Read the model definition and answer for the solid it produces. Units are mm, in the model's axes. Face numbers are marked on the shaded views. A direction names the side the tool comes from. Coordinates: 2 decimals unless noted, no trailing zeros. Loops run counter-clockwise (first coordinate to the right, second up) from the corner with the lowest first, then second, coordinate; pieces in that order, holes last. Notation, with made-up numbers: M -24,-17.75 L 30,-17.75 A28 cw 30,11.25 Z; hole C 52,-19 d6. An arc over 180 degrees is marked long. Put each result on its own line as item: value.
from build123d import *

# Parameters (mm, degrees)
F0_R     = 60
F0_R_2   = 3
F0_R_3   = 15
F0_R_4   = 2
F1_DEPTH = 25


# Not quite as in the source:
# - a feature names something its author has since deleted; it is built from what else it names


with BuildPart() as f1:
    # F0 (on Front) → F1 (new body)
    with BuildSketch(Plane.XZ):
        Circle(F0_R)
        with Locations((-37.5115520048, -38.8443492183)):
            Circle(F0_R_2, mode=Mode.SUBTRACT)
        with BuildLine():
            ThreePointArc((-17.9991214641, -21.8181490168), (-12.909542723, -18.5322896083), (-6.8568272685, -18.7878662921))
            ThreePointArc((-6.8568272685, -18.7878662921), (0.003827401, -19.9999996338), (6.864017636, -18.7852405333))
            ThreePointArc((6.864017636, -18.7852405333), (12.9220689894, -18.5288245474), (18.0146364939, -21.8199476948))
            Line((18.0146364939, -21.8199476948), (27.2720618955, -33.0586128775))
            ThreePointArc((27.2720618955, -33.0586128775), (29.3324432338, -41.5072979988), (23.9974181864, -48.3748273422))
            ThreePointArc((23.9974181864, -48.3748273422), (0, -54), (-23.9974181864, -48.3748273422))
            ThreePointArc((-23.9974181864, -48.3748273422), (-29.3332198415, -41.5036623321), (-27.2673324169, -33.0528755612))
            Line((-27.2673324169, -33.0528755612), (-17.9991214641, -21.8181490168))
        make_face(mode=Mode.SUBTRACT)
        with BuildLine():
            ThreePointArc((-44.5250909536, -30.5534985815), (-45.2912230512, -29.4058687089), (-46.0277820813, -28.2390381684))
            ThreePointArc((-46.0277820813, -28.2390381684), (-46.5604522686, -23.0733436974), (-42.8629692739, -19.4268719232))
            Line((-42.8629692739, -19.4268719232), (-16.9967316552, -10.5409256254))
            ThreePointArc((-16.9967316552, -10.5409256254), (-15.120110809, -11.5154453431), (-15.5299138764, -13.5899226089))
            Line((-15.5299138764, -13.5899226089), (-16.9726013847, -14.8870728677))
            Line((-16.9726013847, -14.8870728677), (-17.1078816805, -15.0240893401))
            Line((-17.1078816805, -15.0240893401), (-35.5662381193, -31.6203804252))
            ThreePointArc((-35.5662381193, -31.6203804252), (-40.2873666152, -33.116567588), (-44.5250909536, -30.5534985815))
        make_face(mode=Mode.SUBTRACT)
        with Locations((-52.3959692189, -13.0637823624)):
            Circle(F0_R_2, mode=Mode.SUBTRACT)
        with Locations((37.5115520048, -38.8443492183)):
            Circle(F0_R_2, mode=Mode.SUBTRACT)
        with BuildLine():
            Line((21.3985322272, -7.6356383993), (45.0061435827, -15.3247300238))
            ThreePointArc((45.0061435827, -15.3247300238), (48.6715278542, -18.6865524369), (48.5414946952, -23.6584719025))
            ThreePointArc((48.5414946952, -23.6584719025), (46.8021183332, -26.9362528857), (44.8417435514, -30.0868415635))
            ThreePointArc((44.8417435514, -30.0868415635), (40.6476491874, -32.6918461445), (35.9197630861, -31.2693239428))
            Line((35.9197630861, -31.2693239428), (17.1994124126, -14.9726488191))
            ThreePointArc((17.1994124126, -14.9726488191), (16.1962922773, -13.1122239789), (16.6688649306, -11.0521012448))
            ThreePointArc((16.6688649306, -11.0521012448), (17.2612476069, -10.1019468943), (17.7995287636, -9.1201302509))
            ThreePointArc((17.7995287636, -9.1201302509), (19.3255292381, -7.7148076154), (21.3985322272, -7.6356383993))
        make_face(mode=Mode.SUBTRACT)
        with Locations((52.3959692189, -13.0637823624)):
            Circle(F0_R_2, mode=Mode.SUBTRACT)
        with BuildLine():
            Line((-14.9909636957, 40.1406403471), (-9.8955105801, 26.4967709421))
            ThreePointArc((-9.8955105801, 26.4967709421), (-9.5946622296, 20.4461367535), (-12.8423558576, 15.3321197499))
            ThreePointArc((-12.8423558576, 15.3321197499), (-18.0436420311, 8.6271074095), (-19.9965959104, 0.3689877998))
            ThreePointArc((-19.9965959104, 0.3689877998), (-22.4237136521, -5.9792994979), (-28.3480846215, -9.3099872294))
            Line((-28.3480846215, -9.3099872294), (-42.3172195747, -11.6422803342))
            ThreePointArc((-42.3172195747, -11.6422803342), (-50.2710809676, -9.5390364788), (-53.9558535504, -2.1830867246))
            ThreePointArc((-53.9558535504, -2.1830867246), (-48.0998424018, 24.5439434672), (-29.8951202889, 44.9697874457))
            ThreePointArc((-29.8951202889, 44.9697874457), (-21.276616009, 46.1551447236), (-14.9909636957, 40.1406403471))
        make_face(mode=Mode.SUBTRACT)
        with BuildLine():
            Line((-4.4279652677, 22.3694685585), (-9.2474940163, 46.7170617057))
            ThreePointArc((-9.2474940163, 46.7170617057), (-8.1285920064, 51.5258593406), (-3.7819096653, 53.8674034949))
            ThreePointArc((-3.7819096653, 53.8674034949), (-0.1220878193, 53.9998619865), (3.5382955571, 53.8839536834))
            ThreePointArc((3.5382955571, 53.8839536834), (7.9230697986, 51.5261035304), (9.0182868498, 46.6695407434))
            Line((9.0182868498, 46.6695407434), (3.9392668723, 22.3644794699))
            ThreePointArc((3.9392668723, 22.3644794699), (2.8434498256, 20.6092434876), (0.8719123918, 19.9809851804))
            ThreePointArc((0.8719123918, 19.9809851804), (-0.2100325239, 19.9988971281), (-1.2913626084, 19.9582660222))
            ThreePointArc((-1.2913626084, 19.9582660222), (-3.31345185, 20.5735591973), (-4.4279652677, 22.3694685585))
        make_face(mode=Mode.SUBTRACT)
        with Locations((-14.8844172141, 51.9081315807)):
            Circle(F0_R_2, mode=Mode.SUBTRACT)
        Circle(F0_R_3, mode=Mode.SUBTRACT)
        with BuildLine():
            ThreePointArc((12.8423558576, 15.3321197499), (9.5946622296, 20.4461367535), (9.8955105801, 26.4967709421))
            Line((9.8955105801, 26.4967709421), (14.9909636957, 40.1406403471))
            ThreePointArc((14.9909636957, 40.1406403471), (21.276616009, 46.1551447236), (29.8951202889, 44.9697874457))
            ThreePointArc((29.8951202889, 44.9697874457), (46.7619600734, 27.0059084294), (53.8916763243, 3.4186580637))
            ThreePointArc((53.8916763243, 3.4186580637), (50.6128315094, -4.6370491105), (42.2649270201, -7.0778956919))
            Line((42.2649270201, -7.0778956919), (27.9019654451, -4.6798491157))
            ThreePointArc((27.9019654451, -4.6798491157), (22.506844055, -1.9164656047), (19.6991831261, 3.4557465422))
            ThreePointArc((19.6991831261, 3.4557465422), (17.3205080757, 10), (12.8423558576, 15.3321197499))
        make_face(mode=Mode.SUBTRACT)
        with Locations((14.8844172141, 51.9081315807)):
            Circle(F0_R_2, mode=Mode.SUBTRACT)
        Circle(F0_R_3)
        with Locations((-5.8778525229, -8.0901699437)):
            Circle(F0_R_4, mode=Mode.SUBTRACT)
        with BuildLine():
            ThreePointArc((-3.8729833462, 1), (-2.8284271247, 2.8284271247), (-1, 3.8729833462))
            Line((-1, 3.8729833462), (-1, 5))
            ThreePointArc((-1, 5), (0, 6), (1, 5))
            Line((1, 5), (1, 3.8729833462))
            ThreePointArc((1, 3.8729833462), (2.8284271247, 2.8284271247), (3.8729833462, 1))
            Line((3.8729833462, 1), (4.9514505081, 1))
            ThreePointArc((4.9514505081, 1), (5.9514505081, 0), (4.9514505081, -1))
            Line((4.9514505081, -1), (3.8729833462, -1))
            ThreePointArc((3.8729833462, -1), (2.8284271247, -2.8284271247), (1, -3.8729833462))
            Line((1, -3.8729833462), (1, -5.0126444548))
            ThreePointArc((1, -5.0126444548), (0, -6.0126444548), (-1, -5.0126444548))
            Line((-1, -5.0126444548), (-1, -3.8729833462))
            ThreePointArc((-1, -3.8729833462), (-2.8284271247, -2.8284271247), (-3.8729833462, -1))
            Line((-3.8729833462, -1), (-5.0453338772, -1))
            ThreePointArc((-5.0453338772, -1), (-6.0453338772, 0), (-5.0453338772, 1))
            Line((-5.0453338772, 1), (-3.8729833462, 1))
        make_face(mode=Mode.SUBTRACT)
        with Locations((5.8778525229, -8.0901699437)):
            Circle(F0_R_4, mode=Mode.SUBTRACT)
        with Locations((-9.510565163, 3.0901699437)):
            Circle(F0_R_4, mode=Mode.SUBTRACT)
        with Locations((9.510565163, 3.0901699437)):
            Circle(F0_R_4, mode=Mode.SUBTRACT)
        with Locations((0, 10)):
            Circle(F0_R_4, mode=Mode.SUBTRACT)
    extrude(amount=F1_DEPTH)


solid = f1.part
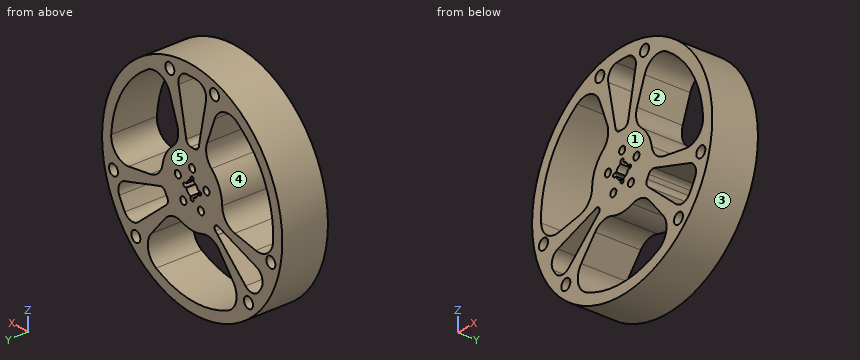
1) Which of the six approach directions +Z, -Z, +X, -X, +Y, -Y give full straight-line access (tool end or side, diameter ignored) to the marked faces 4 and 5?
Answer list:
face 4: +Y, -Y
face 5: +Z, -Z, +X, -X, +Y
2) Determine the mould class of the marked faces 1, 2 and 3 for opening direction X: released by +X, released by -X, zero draft, split by the parting line, or undercut.
Answer list:
face 1: zero draft
face 2: undercut
face 3: split by the parting line
3) Find section A-A, the plane z = 10. Write down the section's boundary in (x, y).
Answer list:
outline: M -59.16,-25 L -53.07,-25 L -53.07,0 L -59.16,0 Z; M -17.32,-25 L -2,-25 L -2,0 L -17.32,0 Z; M 2,-25 L 17.32,-25 L 17.32,0 L 2,0 Z; M 53.07,-25 L 59.16,-25 L 59.16,0 L 53.07,0 Z
4) Given pin 1 Ø1.3 at (y, z) = (-11, -4.5) entering from +X; pin 2 Ø3 at (x, y) = (-27, -21.5) entering from -Z; pin 3 Ø0.6 at (y, z) = (-15, -4.5) entering from -X; pin 4 Ø1 at (x, z) = (-12.5, 14.5) entering from +Y, each flat-ended and moving along its own axis, determine where each tip first touches the part or whether it passes through.
Answer list:
pin 1: stops at x = 59.88
pin 2: stops at z = -54.31
pin 3: stops at x = -59.85
pin 4: stops at y = 0
5) Straight lines are drawn through the part: line 1 (Z direction, x = -15.5, y = -5); line 2 (Z direction, x = 46.5, y = -17.75); line 3 (Z direction, x = 43.5, y = -18.25). For each, find the intervals that lie inside material, in ascending order. Write a range as [from, to].
Answer list:
line 1: z = [-57.96, -51.73], [-19.65, -13.56], [-11, 12.64], [41.28, 48.97], [54.84, 57.96]
line 2: z = [-37.92, -27.45], [-16.05, -6.87], [27.45, 37.92]
line 3: z = [-41.32, -31.51], [-14.83, -7.21], [32, 41.32]
6) Find section B-B, the plane y = -6.5. Count the separate pieces of the cut face and the enclosed holes in it, plus the area to 3 significant figures.
Answer list:
separate pieces: 1
enclosed holes: 18
area: 4,660 mm^2
